Model file for the job. Use its own axes, mm. A direction names the side the tool comes from. Round coordinates to 2 decimals unless told otherwise and drop trailing zeros. Loops run counter-clockwise (first coordinate to the right, second up) from the corner with the lowest first, then second, coordinate; pieces in that order, holes last. Notation, with made-up numbers: (-31, 61.5) - (15, 61.5) arc R27 cw to (15, 86.5) - close; hole circle Ø10 at (26.5, -11.5). An arc over 180 degrees is marked (long way). Answer as a JSON object with one key per item and string values.
from build123d import *

# Parameters (mm, degrees)
F1_DEPTH = 66.548
F0_W     = 10.9235864809
F0_H     = 33.6925396672
F2_DEPTH = 10.922
F4_DEPTH = 10.7584603328
F5_DEPTH = 50.8
F7_DEPTH = 127
F8_DEPTH = 127


with BuildPart() as f1:
    # F0 (on Top) → F1 (new body)
    with BuildSketch(Plane.XY):
        Polygon((37.8037942689, 44.45), (-76.4962057311, 44.45), (-76.4962057311, 33.6925396672), (-65.5726192503, 33.6925396672), (-12.9962057311, 33.6925396672), (37.8037942689, 33.6925396672), align=None)
    extrude(amount=F1_DEPTH)

    # F0 (on Top) → F2 (join)
    with BuildSketch(Plane.XY):
        with Locations((-71.0344124907, 16.8462698336)):
            Rectangle(F0_W, F0_H)
        Polygon((-12.9962057311, 33.6925396672), (-65.5726192503, 33.6925396672), (-65.5726192503, 0), align=None)
    extrude(amount=F2_DEPTH)

    # F3 (on face) → F4 (cut, through all)
    with BuildSketch(Plane.XZ.offset(-33.6925396672)):
        with BuildLine():
            ThreePointArc((26.6277942689, 19.05), (13.1860354738, 24.6177587951), (18.7537942689, 11.176))
            ThreePointArc((18.7537942689, 11.176), (24.3215530639, 13.4822412049), (26.6277942689, 19.05))
        make_face()
    extrude(amount=-F4_DEPTH, mode=Mode.SUBTRACT)

    # F0 (on Top) → F5 (join)
    with BuildSketch(Plane.XY):
        with Locations((-71.0344124907, 16.8462698336)):
            Rectangle(F0_W, F0_H)
    extrude(amount=F5_DEPTH)

    # F6 (on face) → F7 (cut)
    with BuildSketch(Plane.YZ.offset(-65.5726192503)):
        Polygon((0, 50.8), (0, 22.098), (16.5711074263, 50.8), align=None)
    extrude(amount=-F7_DEPTH, mode=Mode.SUBTRACT)

    # F3 (on face) → F8 (cut)
    with BuildSketch(Plane.XZ.offset(-33.6925396672)):
        Polygon((-44.7462057311, 66.548), (37.8037942689, 44.4287941648), (37.8037942689, 66.548), align=None)
    extrude(amount=-F8_DEPTH, mode=Mode.SUBTRACT)


solid = f1.part
1) Drop flat-ended pins along their axis: P1, Ø8.5, axis at x = -72.5, y = 22, coming from the +Z side; P2, Ø1, axis at x = 14, z = 41.5, coming from the -Y side; P3, Ø12, axis at y = 12, z = 31, coming from the +X side. Give the stop position or say it passes through.
Values follow:
{"P1": "z = 50.8", "P2": "y = 33.69", "P3": "x = -65.57"}
2) Slice it at C-C on y = 6. List the corners of the cut face in (x, z), then the cut area to 3 significant figures.
Values follow:
{"outline": "(-76.5, 0) - (-56.21, 0) - (-56.21, 10.92) - (-65.57, 10.92) - (-65.57, 32.49) - (-76.5, 32.49) - close", "area": "457 mm²"}
3) Slice it at D-D on x = -39. List the corners of the cut face in (y, z).
Values follow:
{"outline": "(17.03, 0) - (44.45, 0) - (44.45, 65.01) - (33.69, 65.01) - (33.69, 10.92) - (17.03, 10.92) - close"}
4) Slice it at B-B on z = 25. List the corners of the cut face in (x, y), then the cut area to 3 significant figures.
Values follow:
{"outline": "(-76.5, 1.68) - (-65.57, 1.68) - (-65.57, 33.69) - (13.6, 33.69) - (13.6, 44.45) - (-76.5, 44.45) - close; (23.91, 33.69) - (37.8, 33.69) - (37.8, 44.45) - (23.91, 44.45) - close", "area": "1,470 mm²"}
5) Probe probe 1 along X at (y, z) = (36.25, 19.05); probe 2 along Y at (x, z) = (-21.5, 15.5); probe 3 along X at (y, z) = (31.5, 18). List the from-to ranges inside material, lowest first.
Values follow:
{"probe 1": "-76.5 to 10.88, 26.63 to 37.8", "probe 2": "33.69 to 44.45", "probe 3": "-76.5 to -65.57"}
6) Tool access for faces 1 (the flat face through (-65.573, 20, 31)), 2 (the flat face through (-76.496, 27, 25)), 3 (the flat face through (-71, 25, 50.8)): list every direction of +Z, -Z, +X, -X, +Y, -Y with a clear straight run to the whole face (end or side of a thin tool).
Values follow:
{"face 1": "+Z, +X, -Y", "face 2": "+Z, -Z, -X, +Y, -Y", "face 3": "+Z, +X, -X, -Y"}
7) Slice it at A-A on y = 39.5. List the corners of the cut face in (x, z).
Values follow:
{"outline": "(-76.5, 0) - (37.8, 0) - (37.8, 44.43) - (-44.75, 66.55) - (-76.5, 66.55) - close; hole circle Ø15.75 at (18.75, 19.05)"}
